The listing builds one solid part. Answer for the finished solid, in the listing's coordinates (mm). Face numbers are marked on the shaded views. A direction names the side the tool comes from. Give positions to 0.01 mm unless a question says otherwise; leave off trailing zeros. Write each loop counter-clockwise with the first axis right and the second up, starting at its lowest first coordinate (ties: lowest second). Pieces come first, ordered by that corner, then holes. Notation, with made-up numbers: (44.25, 85.25) - (100.25, 85.25) arc R9 ccw to (100.25, 96.25) - close; hole circle Ø5 at (23, 68). An arc over 180 degrees is marked (long way). Return JSON: item names as keys, results as strings.
from build123d import *

# Parameters (mm, degrees)
F0_W     = 12.7
F0_H     = 101.6
F1_DEPTH = 12.7
F2_R     = 5.08
F3_R     = 3.81
F4_DEPTH = 76.2


with BuildPart() as f1:
    # F0 (on Top) → F1 (new body)
    with BuildSketch(Plane.XY):
        Polygon((-38.1, -63.5), (38.1, -63.5), (73.039025, -63.5), (38.1, 26.026342), (38.1, 63.5), (-38.1, 63.5), (-38.1, 26.026342), (-73.039025, -63.5), align=None)
        Polygon((-63.744396, -57.149999), (-44.450001, -7.710822), (-44.450001, -57.149999), align=None, mode=Mode.SUBTRACT)
        Polygon((44.45, -57.15), (44.45, -7.710819), (63.744397, -57.15), align=None, mode=Mode.SUBTRACT)
        with Locations((-19.05, 0)):
            Rectangle(F0_W, F0_H, mode=Mode.SUBTRACT)
        with Locations((19.05, 0)):
            Rectangle(F0_W, F0_H, mode=Mode.SUBTRACT)
    extrude(amount=F1_DEPTH)

    # F2
    f2_edges = [f1.edges().sort_by_distance(p)[0] for p in [
        (73.039025, -63.5, 6.35),
        (-73.039025, -63.5, 6.35),
    ]]
    fillet(f2_edges, radius=F2_R)

    # F3 (on face) → F4 (cut)
    with BuildSketch(Plane(origin=(-38.1, 0, 0), x_dir=(0, -1, 0), z_dir=(-1, 0, 0))):
        with Locations((-57.429425, 6.35)):
            Circle(F3_R)
    extrude(amount=-F4_DEPTH, mode=Mode.SUBTRACT)


solid = f1.part
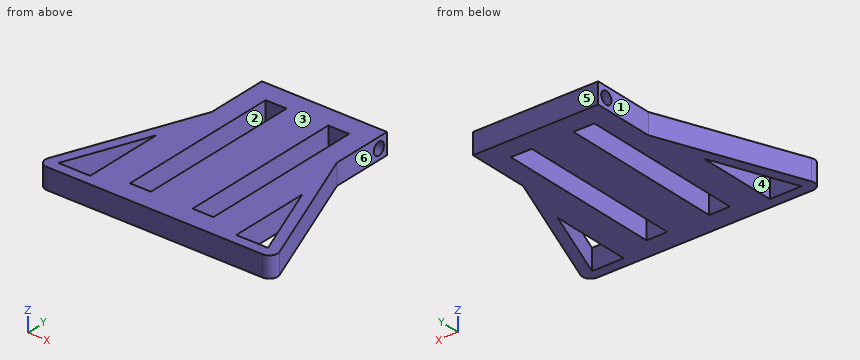
Item 1: A cutting plane is placed at B-B on z = 6.35. Determine the outline of the cut face in (x, y).
Answer below:
{"outline": "(-70.34, -56.57) arc R5.08 ccw to (-65.6, -63.5) - (65.6, -63.5) arc R5.08 ccw to (70.34, -56.57) - (38.1, 26.03) - (38.1, 53.62) - (-38.1, 53.62) - (-38.1, 26.03) - close; (-38.1, 61.24) - (38.1, 61.24) - (38.1, 63.5) - (-38.1, 63.5) - close; hole (-63.74, -57.15) - (-44.45, -57.15) - (-44.45, -7.71) - close; hole (-25.4, -50.8) - (-12.7, -50.8) - (-12.7, 50.8) - (-25.4, 50.8) - close; hole (12.7, -50.8) - (25.4, -50.8) - (25.4, 50.8) - (12.7, 50.8) - close; hole (44.45, -57.15) - (63.74, -57.15) - (44.45, -7.71) - close"}
Item 2: A cutting plane is placed at C-C on y = 8. Determine the outline of the cut face in (x, z), then the cut area to 3 significant figures.
Answer below:
{"outline": "(-45.14, 0) - (-25.4, 0) - (-25.4, 12.7) - (-45.14, 12.7) - close; (-12.7, 0) - (12.7, 0) - (12.7, 12.7) - (-12.7, 12.7) - close; (25.4, 0) - (45.14, 0) - (45.14, 12.7) - (25.4, 12.7) - close", "area": "824 mm²"}
Item 3: Flat-ended cylindrical pins translate along their axes: P1, Ø6.5, axis at y = 52.5, z = 9.5, coming from the +X side; P2, Ø6.5, axis at y = 24.5, z = 8.5, coming from the +X side; P3, Ø6.5, axis at y = -22, z = 6, coming from the +X side. Find the tip coordinate at first contact, or state that the pin passes through.
Answer below:
{"P1": "stops at x = 38.1", "P2": "stops at x = 39.96", "P3": "stops at x = 58.11"}
Item 4: A cutting plane is placed at D-D on x = -60.5. Determine the outline of the cut face in (y, z), then the cut area to 3 significant figures.
Answer below:
{"outline": "(-63.5, 0) - (-57.15, 0) - (-57.15, 12.7) - (-63.5, 12.7) - close; (-48.84, 0) - (-31.37, 0) - (-31.37, 12.7) - (-48.84, 12.7) - close", "area": "302 mm²"}
Item 5: Consider L1, parallel to Y at x = 18.5, z = 6.75; L2, parallel to X at y = 37, z = 2.5; L3, parallel to X at y = -2, z = 10.5. Determine where each line is inside the solid, lowest interval first.
Answer below:
{"L1": "y = -63.5 to -50.8, 50.8 to 53.64, 61.22 to 63.5", "L2": "x = -38.1 to -25.4, -12.7 to 12.7, 25.4 to 38.1", "L3": "x = -49.04 to -25.4, -12.7 to 12.7, 25.4 to 49.04"}
Item 6: For the marked faces 4, 5 and 6, determine the directions among +Z, -Z, +X, -X, +Y, -Y from which every point of the face is accessible in a straight line to the end or side of a thin tool.
Answer below:
{"face 4": "+Z, -Z", "face 5": "+Z, -Z, +X, -X, +Y", "face 6": "+Z, -Z, +X, +Y"}
Item 7: A cutting plane is placed at A-A on x = -15. Determine the outline of the cut face in (y, z).
Answer below:
{"outline": "(-63.5, 0) - (-50.8, 0) - (-50.8, 12.7) - (-63.5, 12.7) - close; (50.8, 0) - (63.5, 0) - (63.5, 12.7) - (50.8, 12.7) - close; hole circle Ø7.62 at (57.43, 6.35)"}
Item 8: The mould has two halves that part along X. Classify the marked faces 1, 2 and 3: +X half, -X half, draft (parallel to the pull), parting line (faces both ways), or undercut.
Answer below:
{"face 1": "-X half", "face 2": "undercut", "face 3": "draft"}
